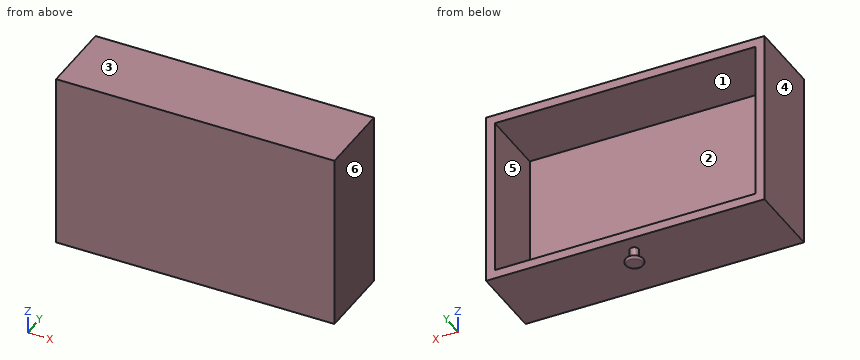
```python
from build123d import *

# Parameters (mm, degrees)
SKETCH1_W           = 475
SKETCH1_H           = 130
BOSS_EXTRUDE1_DEPTH = 300
SHELL1_T            = -15


with BuildPart() as part:
    # Sketch1 → Boss-Extrude1 (new body)
    with BuildSketch(Plane.XY):
        with Locations((186.944444444, 54.744444444)):
            Rectangle(SKETCH1_W, SKETCH1_H)
    extrude(amount=BOSS_EXTRUDE1_DEPTH)

    # Shell1
    shell1_openings = [part.faces().sort_by_distance(p)[0] for p in [
        (186.944444444, 119.744444444, 150),
    ]]
    offset(amount=SHELL1_T, openings=shell1_openings, kind=Kind.INTERSECTION)

    # Sketch3 → Revolve2 (revolve)
    with BuildSketch(Plane.ZY.offset(-186.944444444), mode=Mode.PRIVATE) as revolve2_sk:
        with BuildLine():
            Line((0, 89.744444444), (-25, 89.744444444))
            Line((-25, 89.744444444), (-25, 102.114714247))
            ThreePointArc((-25, 102.114714247), (-22, 105.114714247), (-19, 102.114714247))
            ThreePointArc((-19, 102.114714247), (-17.535533906, 98.579180341), (-14, 97.114714247))
            Line((-14, 97.114714247), (0, 97.114714247))
            Line((0, 97.114714247), (0, 89.744444444))
        make_face()
    revolve(revolve2_sk.sketch.rotate(Axis((186.944444444, 89.744444444, 0), (0, 0, -1)), 90), axis=Axis((186.944444444, 89.744444444, 0), (0, 0, -1)))


solid = part.part
```
Model file for the job. Use its own axes, mm. Face numbers are marked on the shaded views. A direction names the side the tool comes from. Round coordinates to 2 decimals unless told otherwise and drop trailing zeros. Order: outer loops, then holes, each group sorted by start corner. A loop starts at its lowest first (then second) coordinate and runs counter-clockwise, first axis right, second up. Notation, with made-up numbers: M 20.5,83 L 60.5,83 A18 ccw 60.5,116 Z; hole C 80,79 d2. An arc over 180 degrees is marked long. Use CSV: the item, a comma, the result in double quotes.
Item 1: Probe probe 1 along X at (y, z) = (108, 143); probe 2 along Z at (x, y) = (387, 7.5); probe 3 along Y at (x, z) = (356, 78). List the from-to ranges inside material, lowest first.
Worked answers:
probe 1,"-50.56 to -35.56, 409.44 to 424.44"
probe 2,"0 to 15, 285 to 300"
probe 3,"-10.26 to 4.74"
Item 2: Pin check, flat tip, straight feed: pin 1 (8 mm diameter, centred on x = 244.5, z = 29, fed in from +Y). Stop position of the tip, or through.
Worked answers:
pin 1,"y = 4.74"
Item 3: Pull direction Z, two halves, no side cores. Call the marked faces 1, 2, 3 and 4: released by +Z, released by -Z, zero draft, split by the parting line, or undercut.
Worked answers:
face 1,"undercut"
face 2,"undercut"
face 3,"released by +Z"
face 4,"zero draft"
Item 4: Saw through at B-B (x = 56.5). List the corners of the cut face in (y, z), plus the area to 3 significant figures.
Worked answers:
outline,"M -10.26,0 L 119.74,0 L 119.74,15 L 4.74,15 L 4.74,285 L 119.74,285 L 119.74,300 L -10.26,300 Z"
area,"7,950 mm²"
Item 5: Saw through at A-A (y = 29). List the corners of the cut face in (x, z), plus the area to 4 significant figures.
Worked answers:
outline,"M -50.56,0 L 424.44,0 L 424.44,300 L -50.56,300 Z; hole M -35.56,15 L 409.44,15 L 409.44,285 L -35.56,285 Z"
area,"22,350 mm²"
Item 6: Which spindle directions (+Z, -Z, +X, -X, +Y, -Y) get a long thin tool onto all of the face, cutting with end or side? Do the marked faces 5 and 6. Say none if no direction does.
Worked answers:
face 5,"+Y"
face 6,"+Z, -Z, +X, +Y, -Y"
Item 7: Saw through at C-C (z = 79.5). List the corners of the cut face in (x, y).
Worked answers:
outline,"M -50.56,-10.26 L 424.44,-10.26 L 424.44,119.74 L 409.44,119.74 L 409.44,4.74 L -35.56,4.74 L -35.56,119.74 L -50.56,119.74 Z"
